Design review of the part built by this model. Coordinates are the model's own, in mm. Face numbers are marked on the shaded views. A direction names the side the tool comes from. Coordinates: 2 decimals unless noted, no trailing zeros. Loops run counter-clockwise (first coordinate to the right, second up) from the corner with the lowest first, then second, coordinate; pieces in that order, holes last. Notation, with made-up numbers: (35, 41) -> (44, 41) arc R24 ccw to (44, 80) -> close; hole circle Ø1 at (-23, -5). An arc over 180 degrees is marked (long way). Answer as a JSON object with one key per item and string values.
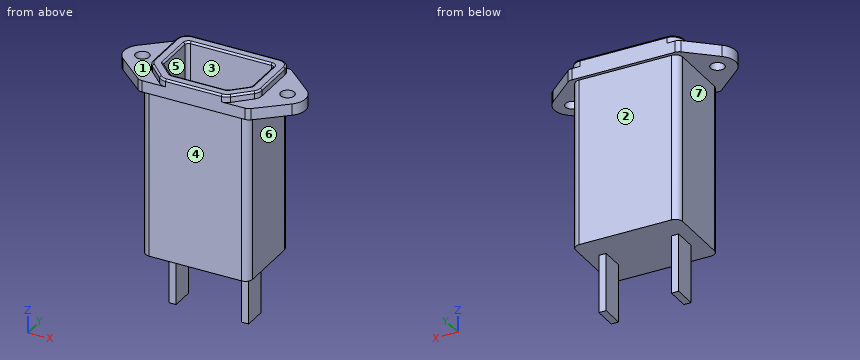
```python
from build123d import *

# Parameters (mm, degrees)
SKETCH1_R           = 1.9
BOSS_EXTRUDE1_DEPTH = 3.15
BOSS_EXTRUDE2_DEPTH = 2
FILLET1_R           = 0.5
BOSS_EXTRUDE3_DEPTH = 46
SKETCH4_W           = 2
SKETCH4_H           = 6.35
BOSS_EXTRUDE4_DEPTH = 16
CUT_EXTRUDE1_START  = -11.1
CUT_EXTRUDE1_DEPTH  = 11.1


with BuildPart() as part:
    # Sketch1 → Boss-Extrude1 (new body)
    with BuildSketch(Plane.XY):
        with BuildLine():
            Line((-15.565068493, 10.506849315), (-23.287671233, 3.767123288))
            ThreePointArc((-23.287671233, 3.767123288), (-25, 0), (-23.287671233, -3.767123288))
            Line((-23.287671233, -3.767123288), (-15.565068493, -10.506849315))
            ThreePointArc((-15.565068493, -10.506849315), (-14.952246883, -10.872658355), (-14.25, -11))
            Line((-14.25, -11), (14.25, -11))
            ThreePointArc((14.25, -11), (14.952246883, -10.872658355), (15.565068493, -10.506849315))
            Line((15.565068493, -10.506849315), (23.287671233, -3.767123288))
            ThreePointArc((23.287671233, -3.767123288), (25, 0), (23.287671233, 3.767123288))
            Line((23.287671233, 3.767123288), (15.565068493, 10.506849315))
            ThreePointArc((15.565068493, 10.506849315), (14.952246883, 10.872658355), (14.25, 11))
            Line((14.25, 11), (-14.25, 11))
            ThreePointArc((-14.25, 11), (-14.952246883, 10.872658355), (-15.565068493, 10.506849315))
        make_face()
        with Locations((-20, 0)):
            Circle(SKETCH1_R, mode=Mode.SUBTRACT)
        with Locations((20, 0)):
            Circle(SKETCH1_R, mode=Mode.SUBTRACT)
        with BuildLine():
            Line((7.342503403, -8.15), (-7.342503403, -8.15))
            ThreePointArc((-7.342503403, -8.15), (-7.719871127, -8.076063497), (-8.041436351, -7.865187202))
            Line((-8.041436351, -7.865187202), (-12.15, -3.85))
            Line((-12.15, -3.85), (-12.15, 7.15))
            ThreePointArc((-12.15, 7.15), (-11.857106781, 7.857106781), (-11.15, 8.15))
            Line((-11.15, 8.15), (11.15, 8.15))
            ThreePointArc((11.15, 8.15), (11.857106781, 7.857106781), (12.15, 7.15))
            Line((12.15, 7.15), (12.15, -3.429037417))
            ThreePointArc((12.15, -3.429037417), (12.071665055, -3.817023919), (11.848932948, -4.144224619))
            Line((11.848932948, -4.144224619), (8.041436351, -7.865187202))
            ThreePointArc((8.041436351, -7.865187202), (7.719871127, -8.076063497), (7.342503403, -8.15))
        make_face(mode=Mode.SUBTRACT)
    extrude(amount=BOSS_EXTRUDE1_DEPTH)

    # Sketch2 → Boss-Extrude2 (add)
    with BuildSketch(Plane.XY.offset(3.15)):
        with BuildLine():
            Line((15, -3.786855613), (15, 8))
            ThreePointArc((15, 8), (14.121320344, 10.121320344), (12, 11))
            Line((12, 11), (-12, 11))
            ThreePointArc((-12, 11), (-14.121320344, 10.121320344), (-15, 8))
            Line((-15, 8), (-15, -3.786855613))
            ThreePointArc((-15, -3.786855613), (-14.764995165, -4.95081512), (-14.096798843, -5.93241722))
            Line((-14.096798843, -5.93241722), (-9.785674354, -10.145561607))
            ThreePointArc((-9.785674354, -10.145561607), (-8.820978681, -10.778190492), (-7.68887551, -11))
            Line((-7.68887551, -11), (7.68887551, -11))
            ThreePointArc((7.68887551, -11), (8.820978681, -10.778190492), (9.785674354, -10.145561607))
            Line((9.785674354, -10.145561607), (14.096798843, -5.93241722))
            ThreePointArc((14.096798843, -5.93241722), (14.764995165, -4.95081512), (15, -3.786855613))
        make_face()
        with BuildLine():
            Line((-8.041436351, -7.865187202), (-12.15, -3.85))
            Line((-12.15, -3.85), (-12.15, 7.15))
            ThreePointArc((-12.15, 7.15), (-11.857106781, 7.857106781), (-11.15, 8.15))
            Line((-11.15, 8.15), (11.15, 8.15))
            ThreePointArc((11.15, 8.15), (11.857106781, 7.857106781), (12.15, 7.15))
            Line((12.15, 7.15), (12.15, -3.429037417))
            ThreePointArc((12.15, -3.429037417), (12.071665055, -3.817023919), (11.848932948, -4.144224619))
            Line((11.848932948, -4.144224619), (8.041436351, -7.865187202))
            ThreePointArc((8.041436351, -7.865187202), (7.719871127, -8.076063497), (7.342503403, -8.15))
            Line((7.342503403, -8.15), (-7.342503403, -8.15))
            ThreePointArc((-7.342503403, -8.15), (-7.719871127, -8.076063497), (-8.041436351, -7.865187202))
        make_face(mode=Mode.SUBTRACT)
    extrude(amount=BOSS_EXTRUDE2_DEPTH)

    # Fillet1
    fillet1_edges = [part.edges().sort_by_distance(p)[0] for p in [
        (-12.15, 1.65, 5.15),
        (-10.095718176, -5.857593601, 5.15),
        (8.820978681, -10.778190492, 5.15),
        (11.941236599, -8.038989413, 5.15),
        (14.764995165, -4.95081512, 5.15),
        (15, 2.106572194, 5.15),
        (14.121320344, 10.121320344, 5.15),
        (0, 11, 5.15),
        (-14.121320344, 10.121320344, 5.15),
        (-15, 2.106572194, 5.15),
        (-14.764995165, -4.95081512, 5.15),
        (-11.941236599, -8.038989413, 5.15),
        (-8.820978681, -10.778190492, 5.15),
        (0, -11, 5.15),
        (-7.719871127, -8.076063497, 5.15),
        (0, -8.15, 5.15),
        (7.719871127, -8.076063497, 5.15),
        (9.945184649, -6.004705911, 5.15),
        (12.071665055, -3.817023919, 5.15),
        (12.15, 1.860481292, 5.15),
        (11.857106781, 7.857106781, 5.15),
        (0, 8.15, 5.15),
        (-11.857106781, 7.857106781, 5.15),
    ]]
    fillet(fillet1_edges, radius=FILLET1_R)

    # Sketch3 → Boss-Extrude3 (add)
    with BuildSketch(Plane(origin=(0, 0, 0), x_dir=(-1, 0, 0), z_dir=(0, 0, -1))):
        with BuildLine():
            Line((12.75, -10.075), (-12.75, -10.075))
            ThreePointArc((-12.75, -10.075), (-14.164213562, -9.489213562), (-14.75, -8.075))
            Line((-14.75, -8.075), (-14.75, 8.075))
            ThreePointArc((-14.75, 8.075), (-14.164213562, 9.489213562), (-12.75, 10.075))
            Line((-12.75, 10.075), (12.75, 10.075))
            ThreePointArc((12.75, 10.075), (14.164213562, 9.489213562), (14.75, 8.075))
            Line((14.75, 8.075), (14.75, -8.075))
            ThreePointArc((14.75, -8.075), (14.164213562, -9.489213562), (12.75, -10.075))
        make_face()
    extrude(amount=BOSS_EXTRUDE3_DEPTH)

    # Sketch4 → Boss-Extrude4 (add)
    with BuildSketch(Plane(origin=(0, 0, -46), x_dir=(-1, 0, 0), z_dir=(0, 0, -1))):
        with Locations((-10, 0)):
            Rectangle(SKETCH4_W, SKETCH4_H)
        with Locations((10, 0)):
            Rectangle(SKETCH4_W, SKETCH4_H)
    extrude(amount=BOSS_EXTRUDE4_DEPTH)

    # Sketch5 → Cut-Extrude1 (cut)
    with BuildSketch(Plane.XY.offset(CUT_EXTRUDE1_START)):
        with BuildLine():
            Line((-12.15, 7.15), (-12.15, -3.85))
            Line((-12.15, -3.85), (-8.041436351, -7.865187202))
            ThreePointArc((-8.041436351, -7.865187202), (-7.719871127, -8.076063497), (-7.342503403, -8.15))
            Line((-7.342503403, -8.15), (7.342503403, -8.15))
            ThreePointArc((7.342503403, -8.15), (7.719871127, -8.076063497), (8.041436351, -7.865187202))
            Line((8.041436351, -7.865187202), (11.848932948, -4.144224619))
            ThreePointArc((11.848932948, -4.144224619), (12.071665055, -3.817023919), (12.15, -3.429037417))
            Line((12.15, -3.429037417), (12.15, 7.15))
            ThreePointArc((12.15, 7.15), (11.857106781, 7.857106781), (11.15, 8.15))
            Line((11.15, 8.15), (-11.15, 8.15))
            ThreePointArc((-11.15, 8.15), (-11.857106781, 7.857106781), (-12.15, 7.15))
        make_face()
    extrude(amount=CUT_EXTRUDE1_DEPTH, mode=Mode.SUBTRACT)


solid = part.part
```
1) Clearance check with flat-ended pins moving along their axes: pin 1 Ø5.5 at (y, z) = (0, -4.5) entering from -X; pin 2 Ø5 at (x, y) = (-20, -5) entering from +Z; pin 3 Ø8 at (x, z) = (9, -52) entering from -Y (3 decimals). State where each tip first meets the part, or that it passes through.
Completed:
{"pin 1": "x = -14.75", "pin 2": "z = 3.15", "pin 3": "y = -3.175"}
2) The part is to be moulded in two halves that separate along Y. For the marked faces 1, 2, 3 and 4, say which applies: pulls with the +Y half, pulls with the -Y half, needs draft (parallel to the pull), parting line crosses it, or undercut.
Completed:
{"face 1": "needs draft", "face 2": "pulls with the +Y half", "face 3": "undercut", "face 4": "pulls with the -Y half"}
3) Add section A-A, the plane x = 0.5. Give the boundary of the cut face in (y, z) (3 decimals).
Completed:
{"outline": "(-11, 0) -> (-10.075, 0) -> (-10.075, -46) -> (10.075, -46) -> (10.075, 0) -> (11, 0) -> (11, 4.65) arc R0.5 ccw to (10.5, 5.15) -> (8.65, 5.15) arc R0.5 ccw to (8.15, 4.65) -> (8.15, -11.1) -> (-8.15, -11.1) -> (-8.15, 4.65) arc R0.5 ccw to (-8.65, 5.15) -> (-10.5, 5.15) arc R0.5 ccw to (-11, 4.65) -> close"}
4) Add section C-C, the plane y = 0. Count the separate pieces of the cut face and the enclosed holes in it, and give its area (3 significant figures).
Completed:
{"separate pieces": "3", "enclosed holes": "0", "area": "1,220 mm²"}
5) For the marked faces 5, 6 and 7, list the 3-axis set-ups (+Z, -Z, +X, -X, +Y, -Y) from which the entire face can be reached by the end or side of a thin tool; tool diameter is ignored.
Completed:
{"face 5": "+Z", "face 6": "-Z, +X, +Y, -Y", "face 7": "-Z, -X, +Y, -Y"}
6) Wall thickness on probe 1 along Y at (x, z) = (-1, -1.5) (3 decimals); probe 2 along X at (y, z) = (2, -8.5); probe 3 along Z at (x, y) = (-8, 0.25): over which ranges is each line inside the solid? List them lowest first.
Completed:
{"probe 1": "-10.075 to -8.15, 8.15 to 10.075", "probe 2": "-14.75 to -12.15, 12.15 to 14.75", "probe 3": "-46 to -11.1"}
7) Add section D-D, the plane x = 21. Give the boundary of the cut face in (y, z), and give its area (3 significant figures).
Completed:
{"outline": "(-5.76, 0) -> (-1.62, 0) -> (-1.62, 3.15) -> (-5.76, 3.15) -> close; (1.62, 0) -> (5.76, 0) -> (5.76, 3.15) -> (1.62, 3.15) -> close", "area": "26.1 mm²"}
